The model under review builds one solid part; all positions refer to its coordinate system, in mm. Face numbers are marked on the shaded views. Round coordinates to 2 decimals unless told otherwise and drop trailing zeros. Loops run counter-clockwise (first coordinate to the right, second up) from the corner with the lowest first, then second, coordinate; pieces in that order, holes last. Notation, with made-up numbers: M -35,77.25 L 10,77.25 A10 ccw 10,96.25 Z; hole C 70,34.25 d2. An arc over 180 degrees is marked long. Return JSON: item names as keys, results as strings. Group by question number.
Q1. Consider section D-D (z = 0). State the section outline as (x, y) points, and give its area (3 significant figures).
Q2. To check wall thickness, follow line 1 along X through (y, z) = (4.5, -5); line 2 along X through (y, z) = (6.5, 4.5); line 3 along Z through (x, y) = (-15, 4). State the ranges of each line that lie inside material, in increasing order.
Q3. Consider section A-A (x = 17). State the section outline as (y, z) points, and give its area (3 significant figures).
Q4. Consider section C-C (x = -6.5). State the section outline as (y, z) points.
Q5. Clearance check with flat-ended pins moving along their axes: pin 1 Ø1.5 at (y, z) = (1.5, -14) entering from +X; pin 2 Ø1 at (y, z) = (1.5, 14.5) entering from -X. State where each tip first meets the part, or that it passes through.
Q6. Draft analysis for pull direction X (two halves, no side actions). For the marked faces 1, 2 and 3, state which applies: pulls with the +X half, pulls with the -X half, needs draft (parallel to the pull), parting line crosses it, or undercut.
Q7. Consider section B-B (z = 9.5). State the section outline as (x, y) points, and give its area (3 significant figures).
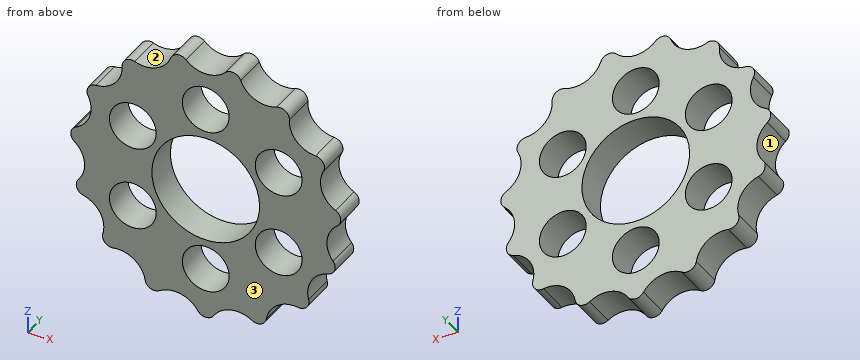
from build123d import *

# Parameters (mm, degrees)
BOSS_EXTRUDE1_DEPTH = 7
SKETCH2_R           = 5
SKETCH2_R_2         = 11.5
CUT_EXTRUDE1_DEPTH  = 42.502327226


with BuildPart() as part:
    # Sketch1 → Boss-Extrude1 (new body)
    with BuildSketch(Plane(origin=(0, 0, 0), x_dir=(1, 0, 0), z_dir=(0, 1, 0))):
        with BuildLine():
            ThreePointArc((1.682317925, 28.081575887), (0, 29), (-1.682317925, 28.081575887))
            ThreePointArc((-1.682317925, 28.081575887), (-5.420186592, 25.49997304), (-9.884932009, 26.33805644))
            ThreePointArc((-9.884932009, 26.33805644), (-11.795362649, 26.492818272), (-12.958679807, 24.969535749))
            ThreePointArc((-12.958679807, 24.969535749), (-15.323360273, 21.090796041), (-19.742987398, 20.040447761))
            ThreePointArc((-19.742987398, 20.040447761), (-21.551199939, 19.404787584), (-21.994368225, 17.540036039))
            ThreePointArc((-21.994368225, 17.540036039), (-22.576985755, 13.034828803), (-26.187300906, 10.277663603))
            ThreePointArc((-26.187300906, 10.277663603), (-27.580638973, 8.961492837), (-27.227030564, 7.077704752))
            ThreePointArc((-27.227030564, 7.077704752), (-25.926845294, 2.725021248), (-28.103592183, -1.262221962))
            ThreePointArc((-28.103592183, -1.262221962), (-28.841134966, -3.031325435), (-27.751891968, -4.608425985))
            ThreePointArc((-27.751891968, -4.608425985), (-24.793717744, -8.055967238), (-25.160517059, -12.583857883))
            ThreePointArc((-25.160517059, -12.583857883), (-25.11473671, -14.5), (-23.478199133, -15.497718004))
            ThreePointArc((-23.478199133, -15.497718004), (-19.373531152, -17.444005802), (-17.866959959, -21.729630455))
            ThreePointArc((-17.866959959, -21.729630455), (-17.045772316, -23.461492837), (-15.144912376, -23.707313787))
            ThreePointArc((-15.144912376, -23.707313787), (-10.603485021, -23.815817289), (-7.484043166, -27.118152514))
            ThreePointArc((-7.484043166, -27.118152514), (-6.029439034, -28.366280421), (-4.192932681, -27.817699643))
            ThreePointArc((-4.192932681, -27.817699643), (0, -26.069657606), (4.192932681, -27.817699643))
            ThreePointArc((4.192932681, -27.817699643), (6.029439034, -28.366280421), (7.484043166, -27.118152514))
            ThreePointArc((7.484043166, -27.118152514), (10.603485021, -23.815817289), (15.144912376, -23.707313787))
            ThreePointArc((15.144912376, -23.707313787), (17.045772316, -23.461492837), (17.866959959, -21.729630455))
            ThreePointArc((17.866959959, -21.729630455), (19.373531152, -17.444005802), (23.478199133, -15.497718004))
            ThreePointArc((23.478199133, -15.497718004), (25.11473671, -14.5), (25.160517059, -12.583857883))
            ThreePointArc((25.160517059, -12.583857883), (24.793717744, -8.055967238), (27.751891968, -4.608425985))
            ThreePointArc((27.751891968, -4.608425985), (28.841134966, -3.031325435), (28.103592183, -1.262221962))
            ThreePointArc((28.103592183, -1.262221962), (25.926845294, 2.725021248), (27.227030564, 7.077704752))
            ThreePointArc((27.227030564, 7.077704752), (27.580638973, 8.961492837), (26.187300906, 10.277663603))
            ThreePointArc((26.187300906, 10.277663603), (22.576985755, 13.034828803), (21.994368225, 17.540036039))
            ThreePointArc((21.994368225, 17.540036039), (21.551199939, 19.404787584), (19.742987398, 20.040447761))
            ThreePointArc((19.742987398, 20.040447761), (15.323360273, 21.090796041), (12.958679807, 24.969535749))
            ThreePointArc((12.958679807, 24.969535749), (11.795362649, 26.492818272), (9.884932009, 26.33805644))
            ThreePointArc((9.884932009, 26.33805644), (5.420186592, 25.49997304), (1.682317925, 28.081575887))
        make_face()
    extrude(amount=BOSS_EXTRUDE1_DEPTH)

    # Sketch2 → Cut-Extrude1 (cut, through all)
    with BuildSketch(Plane(origin=(0, 7, 0), x_dir=(1, 0, 0), z_dir=(0, 1, 0))):
        with Locations(Location((0, 18, 0), (0, 0, 270))):
            Circle(SKETCH2_R)
        with Locations(Location((0, 0, 0), (0, 0, 270))):
            Circle(SKETCH2_R_2)
        with Locations(Location((-15.588457268, -9, 0), (0, 0, 270))):
            Circle(SKETCH2_R)
        with Locations(Location((0, -18, 0), (0, 0, 270))):
            Circle(SKETCH2_R)
        with Locations(Location((15.588457268, -9, 0), (0, 0, 270))):
            Circle(SKETCH2_R)
        with Locations(Location((15.588457268, 9, 0), (0, 0, 270))):
            Circle(SKETCH2_R)
        with Locations(Location((-15.588457268, 9, 0), (0, 0, 270))):
            Circle(SKETCH2_R)
    extrude(amount=-CUT_EXTRUDE1_DEPTH, mode=Mode.SUBTRACT)


solid = part.part
Values:
{
 "1": {"outline": "M -26.93,0 L -11.5,0 L -11.5,7 L -26.93,7 Z; M 11.5,0 L 26.93,0 L 26.93,7 L 11.5,7 Z", "area": "216 mm2"},
 "2": {"line 1": "x = -26.13 to -18.59, -12.59 to -10.36, 10.36 to 12.59, 18.59 to 26.13", "line 2": "x = -27.94 to -17.77, -13.41 to -10.58, 10.58 to 13.41, 17.77 to 27.94", "line 3": "z = -21.34 to -13.97, -4.03 to 4.03, 13.97 to 23.65"},
 "3": {"outline": "M 0,-20.24 L 7,-20.24 L 7,-13.8 L 0,-13.8 Z; M 0,-4.2 L 7,-4.2 L 7,4.2 L 0,4.2 Z; M 0,13.8 L 7,13.8 L 7,23.49 L 0,23.49 Z", "area": "172 mm2"},
 "4": {"outline": "M 0,-25.37 L 7,-25.37 L 7,-9.49 L 0,-9.49 Z; M 0,9.49 L 7,9.49 L 7,28.2 L 0,28.2 Z"},
 "5": {"pin 1": "stops at x = 22.46", "pin 2": "stops at x = -25.32"},
 "6": {"face 1": "pulls with the -X half", "face 2": "undercut", "face 3": "needs draft"},
 "7": {"outline": "M -24.52,0 L -20.56,0 L -20.56,7 L -24.52,7 Z; M -10.61,0 L -6.48,0 L -6.48,7 L -10.61,7 Z; M 6.48,0 L 10.61,0 L 10.61,7 L 6.48,7 Z; M 20.56,0 L 24.52,0 L 24.52,7 L 20.56,7 Z", "area": "113 mm2"}
}
